Geometry: final body of the model. Coordinates: model frame, mm. Face numbers are marked on the shaded views. Give positions to 0.01 mm unless a question says otherwise; leave off trailing zeros. Order: outer loops, then holes, each group sorted by start corner. A loop starts at its lowest first (then second) coordinate and runs counter-clockwise, first axis right, second up. Notation, with made-up numbers: (76.25, 5) -> (126.25, 5) arc R21 cw to (126.25, 18) -> close; hole circle Ø2 at (-13.75, -10.75). An arc over 180 degrees is marked (long way). Answer in a Markdown table with one row per item. Add a question column.
Q1. Cut plane A-A on x = 19.5. Return the cut outline in (y, z).
Q2. Pull-direction query (Y, two-part tool) for the marked faces 1, 2 and 3; classes: +Y half, -Y half, draft (parallel to the pull), parting line (faces both ways), or undercut.
Q3. Cut plane D-D on y = -28. Return the cut outline in (x, z), and give its area (3 significant figures).
Q4. Cut plane C-C on y = 63. Return the cut outline in (x, z), and give its area (4 significant figures).
Q5. Cut plane B-B on z = 12. Return the cut outline in (x, y) (3 decimals).
Q6. Contact query for flat-ended pins moving along their axis: P1, Ø3.5, axis at x = -76.375, y = 0, coming from the -Z side; P2, Ø7, axis at y = 44.5, z = 8, coming from the +X side; P3, Ø4.5, axis at x = -76.5, y = 70.25, coming from the +Z side; P4, Ø2.5, axis at x = -35.5, y = 72.5, coming from the -Z side. Output: stop coordinate, or through.
Q7. Line query: line 1 along Y through (x, z) = (-76.5, 7.25); line 2 along X through (y, z) = (-70.25, 5.25); line 3 along Y through (x, z) = (75.5, 5). Output: solid intervals per line, ascending. Write a range as from..to.
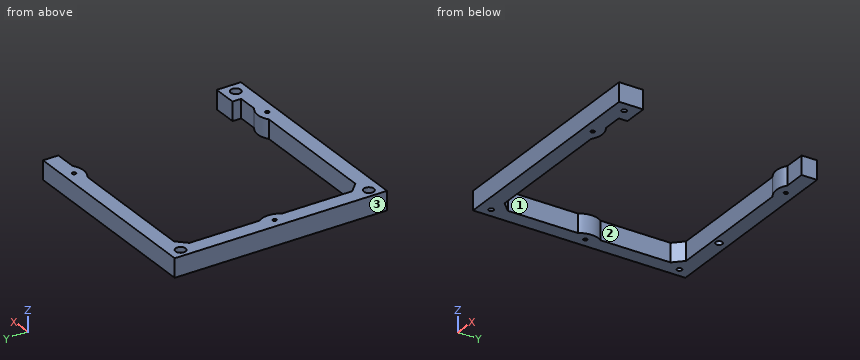
Autodesk Inventor part; units mm, degrees
ref_plane "YZ Plane" through (0, 0, 0) normal (1, 0, 0) x (0, 1, 0)
ref_plane "XZ Plane" through (0, 0, 0) normal (0, 1, 0) x (-1, 0, 0)
ref_plane "XY Plane" through (0, 0, 0) normal (0, 0, 1) x (1, 0, 0)
sketch "Náčrt1" plane through (0, 0, 0) normal (0, 0, 1) x (1, 0, 0)
  line L0 (0, 110.95) -> (0, -110.95)
  line L1 (-116.9, 0) -> (116.9, 0)
  line L2 (67, 79.25) -> (-83.5, 79.25)
  line L3 (-83.5, 79.25) -> (-83.5, -79.25)
  line L4 (-83.5, -79.25) -> (83.5, -79.25)
  line L5 (83.5, -79.25) -> (83.5, -61.25)
  line L6 (83.5, -61.25) -> (65.5, -61.25)
  line L7 (65.5, -61.25) -> (65.5, -67.75)
  line L8 (65.5, -67.75) -> (-72, -67.75)
  line L9 (-72, -67.75) -> (-72, 67.75)
  line L10 (-72, 67.75) -> (67, 67.75)
  line L11 (67, 67.75) -> (67, 79.25)
  arc A0 (-72, -8.415) -> (-72, 8.415) centre (-83.5, 0) ccw
  arc A1 (33.935, 67.75) -> (50.765, 67.75) centre (42.35, 79.25) ccw
  arc A2 (50.765, -67.75) -> (33.935, -67.75) centre (42.35, -79.25) ccw
  point P0 (0, 0)
  dimension "d0" = 11.5
  dimension "d1" = 11.5
  dimension "d2" = 11.5
  dimension "d3" = 150.5
  dimension "d4" = 158.5
  dimension "d5" = 167
  dimension "d6" = 18
  dimension "d7" = 18
  dimension "d8" = 83.5
  dimension "d32" = 28.5
  dimension "d33" = 28.5
  dimension "d35" = 42.35
  dimension "d36" = 42.35
  dimension "d37" = 14.25
extrude "Vysunutí1" add sketch "Náčrt1" along normal blind 14 contours L2 L11 L10 L0 | L0 L10 L9 L1 L3 L2 | L10 A1 | L1 L9 L8 L0 L4 L3 | L8 L7 L6 L5 L4 L0 | A0 L9 L1 | L1 L9 A0 | A2 L8
chamfer "Zkosení1" distance 7 angle 45 2 edges at (-72, 67.75, 7) (-72, -67.75, 7)
sketch "Náčrt2" plane through (0, 0, 14) normal (0, 0, 1) x (1, 0, 0)
  line L0 (67, 79.25) -> (-83.5, 79.25)
  line L1 (-83.5, 79.25) -> (-83.5, -79.25)
  line L2 (-83.5, -79.25) -> (83.5, -79.25)
  line L3 (83.5, -79.25) -> (83.5, -61.25)
  line L4 (83.5, -61.25) -> (65.5, -61.25)
  line L5 (65.5, -61.25) -> (65.5, -67.75)
  line L6 (65.5, -67.75) -> (50.765, -67.75)
  line L7 (-72, -60.75) -> (-65, -67.75)
  line L8 (-72, -60.75) -> (-72, -8.415)
  line L9 (-65, 67.75) -> (-72, 60.75)
  line L10 (-65, 67.75) -> (33.935, 67.75)
  line L11 (67, 67.75) -> (67, 79.25)
  line L12 (0, 110.95) -> (0, -110.95)
  line L13 (-116.9, 0) -> (116.9, 0)
  circle A0 centre (-76.5, 70.25) radius 3.75
  circle A1 centre (-76.5, -70.25) radius 3.75
  circle A2 centre (75.5, -70.25) radius 3.75
  arc A3 (50.765, -67.75) -> (33.935, -67.75) centre (42.35, -79.25) ccw
  line L14 (33.935, -67.75) -> (-65, -67.75)
  arc A4 (-72, -8.415) -> (-72, 8.415) centre (-83.5, 0) ccw
  line L15 (-72, 8.415) -> (-72, 60.75)
  arc A5 (33.935, 67.75) -> (50.765, 67.75) centre (42.35, 79.25) ccw
  line L16 (50.765, 67.75) -> (67, 67.75)
  point P0 (0, 0)
  dimension "d14" = 7.5
  dimension "d15" = 7.5
  dimension "d16" = 7.5
  dimension "d17" = 9
  dimension "d18" = 9
  dimension "d19" = 9
  dimension "d20" = 7
  dimension "d21" = 7
  dimension "d22" = 8
extrude "Vysunutí2" cut sketch "Náčrt2" against normal blind 4 contours A0 | A1 | A2
sketch "Náčrt3" plane through (-76.5, 70.25, 10) normal (0, 0, 1) x (1, 0, 0)
  circle A0 centre (0, 0) radius 3.75
  circle A1 centre (0, -140.5) radius 3.75
  circle A2 centre (152, -140.5) radius 3.75
  circle A3 centre (0, 0) radius 3.75
  point P0 (76.5, -70.25)
hole "Díra1" at (-76.5, 70.25, 10) at (-76.5, -70.25, 10) at (75.5, -70.25, 10) direction (0, 0, -1) diameter 3.7 end through all
sketch "Náčrt4" plane through (0, 0, 0) normal (0, 0, -1) x (-1, 0, 0)
  circle A0 centre (76.5, -70.25) radius 1.85
  circle A1 centre (76.5, 70.25) radius 1.85
  circle A2 centre (-75.5, -70.25) radius 1.85
  line L0 (-67, 79.25) -> (83.5, 79.25)
  line L1 (-67, 67.75) -> (-67, 79.25)
  line L2 (-50.765, 67.75) -> (-67, 67.75)
  arc A3 (-50.765, 67.75) -> (-33.935, 67.75) centre (-42.35, 79.25) ccw
  line L3 (65, 67.75) -> (-33.935, 67.75)
  line L4 (72, 60.75) -> (65, 67.75)
  line L5 (72, 8.415) -> (72, 60.75)
  arc A4 (72, 8.415) -> (72, -8.415) centre (83.5, 0) ccw
  line L6 (72, -60.75) -> (72, -8.415)
  line L7 (65, -67.75) -> (72, -60.75)
  line L8 (-33.935, -67.75) -> (65, -67.75)
  arc A5 (-33.935, -67.75) -> (-50.765, -67.75) centre (-42.35, -79.25) ccw
  line L9 (-65.5, -67.75) -> (-50.765, -67.75)
  line L10 (-65.5, -61.25) -> (-65.5, -67.75)
  line L11 (-83.5, -61.25) -> (-65.5, -61.25)
  line L12 (-83.5, -79.25) -> (-83.5, -61.25)
  line L13 (83.5, -79.25) -> (-83.5, -79.25)
  line L14 (83.5, 79.25) -> (83.5, -79.25)
  line L15 (0, -110.95) -> (0, 110.95)
  line L16 (-116.9, 0) -> (116.9, 0)
  point P0 (0, 0)
  point P1 (34.5, 72.45)
  dimension "d38" = 49
  dimension "d39" = 6.8
hole "Díra2" at (-34.5, 72.45, 0) direction (0, 0, 1) diameter 5 depth 4.3
sketch "Náčrt5" plane through (0, 0, 14) normal (0, 0, 1) x (1, 0, 0)
  arc A0 (33.935, 67.75) -> (50.765, 67.75) centre (42.35, 79.25) ccw
  arc A1 (-72, -8.415) -> (-72, 8.415) centre (-83.5, 0) ccw
  arc A2 (50.765, -67.75) -> (33.935, -67.75) centre (42.35, -79.25) ccw
  line L0 (-116.9, 0) -> (116.9, 0)
  line L1 (0, 110.95) -> (0, -110.95)
  circle A3 centre (75.5, -70.25) radius 3.75
  circle A4 centre (-76.5, -70.25) radius 3.75
  circle A5 centre (-76.5, 70.25) radius 3.75
  line L2 (67, 79.25) -> (-83.5, 79.25)
  line L3 (-83.5, 79.25) -> (-83.5, -79.25)
  line L4 (-83.5, -79.25) -> (83.5, -79.25)
  line L5 (83.5, -79.25) -> (83.5, -61.25)
  line L6 (83.5, -61.25) -> (65.5, -61.25)
  line L7 (65.5, -61.25) -> (65.5, -67.75)
  line L8 (65.5, -67.75) -> (50.765, -67.75)
  arc A6 (50.765, -67.75) -> (33.935, -67.75) centre (42.35, -79.25) ccw
  line L9 (33.935, -67.75) -> (-65, -67.75)
  line L10 (-72, -60.75) -> (-65, -67.75)
  line L11 (-72, -60.75) -> (-72, -8.415)
  arc A7 (-72, -8.415) -> (-72, 8.415) centre (-83.5, 0) ccw
  line L12 (-72, 8.415) -> (-72, 60.75)
  line L13 (-65, 67.75) -> (-72, 60.75)
  line L14 (-65, 67.75) -> (33.935, 67.75)
  arc A8 (33.935, 67.75) -> (50.765, 67.75) centre (42.35, 79.25) ccw
  line L15 (50.765, 67.75) -> (67, 67.75)
  line L16 (67, 67.75) -> (67, 79.25)
  point P0 (0, 0)
  point P1 (-76.375, 0)
  point P2 (42.35, 72.125)
  point P3 (42.35, -72.125)
  dimension "d47" = 7.125
  dimension "d48" = 42.35
  dimension "d49" = 7.125
  dimension "d50" = 42.35
  dimension "d51" = 7.125
hole "Díra3" at (-76.375, 0, 14) at (42.35, 72.125, 14) at (42.35, -72.125, 14) direction (0, 0, -1) diameter 2.8 depth 14
properties part number "display_cover_part2" material "Polystyren"
Completed:
| question | item | result |
|---|---|---|
| 1 | outline | (-79.25, 0) -> (-67.75, 0) -> (-67.75, 14) -> (-79.25, 14) -> close; (67.75, 0) -> (79.25, 0) -> (79.25, 14) -> (67.75, 14) -> close |
| 2 | face 1 | undercut |
| 2 | face 2 | undercut |
| 2 | face 3 | draft |
| 3 | outline | (-83.5, 0) -> (-72, 0) -> (-72, 14) -> (-83.5, 14) -> close |
| 3 | area | 161 mm² |
| 4 | outline | (-83.5, 0) -> (-69.75, 0) -> (-69.75, 14) -> (-83.5, 14) -> close |
| 4 | area | 192.5 mm² |
| 5 | outline | (-83.5, -79.25) -> (83.5, -79.25) -> (83.5, -61.25) -> (65.5, -61.25) -> (65.5, -67.75) -> (50.765, -67.75) arc R14.25 ccw to (33.935, -67.75) -> (-65, -67.75) -> (-72, -60.75) -> (-72, -8.415) arc R14.25 ccw to (-72, 8.415) -> (-72, 60.75) -> (-65, 67.75) -> (33.935, 67.75) arc R14.25 ccw to (50.765, 67.75) -> (67, 67.75) -> (67, 79.25) -> (-83.5, 79.25) -> close; hole circle Ø7.5 at (-76.5, -70.25); hole circle Ø7.5 at (-76.5, 70.25); hole circle Ø2.8 at (-76.375, 0); hole circle Ø2.8 at (42.35, -72.125); hole circle Ø2.8 at (42.35, 72.125); hole circle Ø7.5 at (75.5, -70.25) |
| 6 | P1 | stops at z = 0 |
| 6 | P2 | stops at x = -72 |
| 6 | P3 | stops at z = 10 |
| 6 | P4 | stops at z = 4.3 |
| 7 | line 1 | y = -79.25..-72.1, -68.4..-1.39, 1.39..68.4, 72.1..79.25 |
| 7 | line 2 | x = -83.5..-78.35, -74.65..73.65, 77.35..83.5 |
| 7 | line 3 | y = -79.25..-72.1, -68.4..-61.25 |
